Design review of the part shown in the three views and the two pictorial views. Dimensions are in mm from the part's minimum x, y and z. Give positions to 0.01 mm unless a question says otherwise; leave off trailing zeros. Order: outer loops, then holes, each group sorted by start corner. A loop starts at its lowest first (then second) coordinate and runs counter-clockwise, first axis right, second up.
Item 1: For probe 1 along Z at (x, y) = (128, 1.1) (1 decimal); probe 2 along X at (y, z) = (2.05, 65.5); probe 3 along X at (y, z) = (2.65, 12) (1 decimal), list the stretches that pass through material, from the lowest coordinate up.
Item 2: Consider section A-A (z = 64.77). Give the boundary of the cut face in (x, y).
Item 3: For P1, Ø10, axis at x = 47, z = 7.5, coming from the -Y side; P2, Ø4, axis at x = 14.732, z = 10.287, coming from the +Y side, all flat-tipped, find the tip position at first contact; note any pin that passes through.
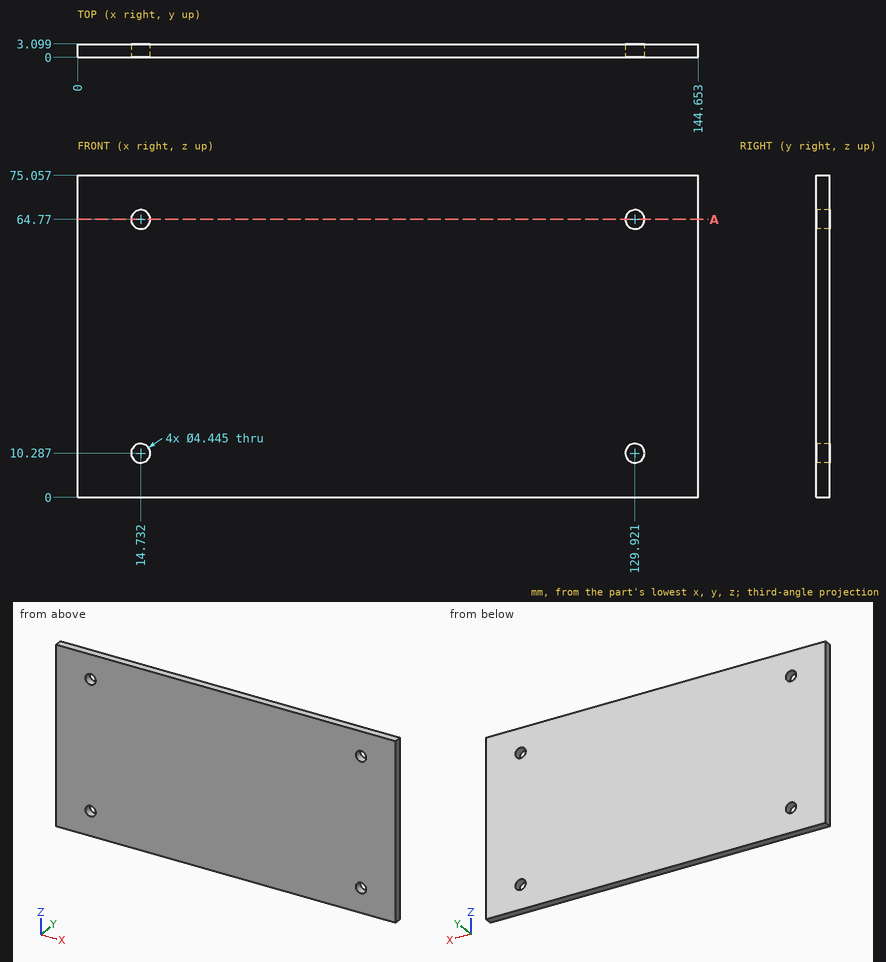
Resolved:
1. probe 1: z = 0 to 9.2, 11.4 to 63.7, 65.9 to 75.1
1. probe 2: x = 0 to 12.63, 16.83 to 127.82, 132.02 to 144.65
1. probe 3: x = 0 to 13.3, 16.1 to 128.5, 131.3 to 144.7
2. outline: (0, 0) - (12.51, 0) - (12.51, 3.1) - (0, 3.1) - close; (16.95, 0) - (127.7, 0) - (127.7, 3.1) - (16.95, 3.1) - close; (132.14, 0) - (144.65, 0) - (144.65, 3.1) - (132.14, 3.1) - close
3. P1: stops at y = 0
3. P2: passes through
